The listing builds one solid part. Answer for the finished solid, in the listing's coordinates (mm). A direction names the side the tool comes from. Coordinates: 2 decimals unless noted, no trailing zeros. Loops run counter-clockwise (first coordinate to the right, second up) from the corner with the lowest first, then second, coordinate; pieces in that order, holes last. Notation, with made-up numbers: (53, 87) - (97, 87) arc R38 ccw to (97, 125) - close; hole circle Ø7 at (26.5, -6.5). An arc over 180 degrees is marked (long way). One line per question, with ' | ' between items.
from build123d import *

# Parameters (mm, degrees)
F0_W     = 396.875
F0_H     = 193.675
F1_DEPTH = 193.675
F3_DEPTH = 396.875
F5_R     = 1.45288
F6_DEPTH = 161.925


with BuildPart() as f1:
    # F0 (on Top) → F1 (new body)
    with BuildSketch(Plane.XY):
        with Locations((198.4375, -96.8375)):
            Rectangle(F0_W, F0_H)
        with BuildLine():
            ThreePointArc((31.75, -50.8), (37.329616, -37.329616), (50.8, -31.75))
            Line((50.8, -31.75), (166.6875, -31.75))
            ThreePointArc((166.6875, -31.75), (180.157884, -37.329616), (185.7375, -50.8))
            Line((185.7375, -50.8), (185.7375, -142.875))
            ThreePointArc((185.7375, -142.875), (180.157884, -156.345384), (166.6875, -161.925))
            Line((166.6875, -161.925), (50.8, -161.925))
            ThreePointArc((50.8, -161.925), (37.329616, -156.345384), (31.75, -142.875))
            Line((31.75, -142.875), (31.75, -50.8))
        make_face(mode=Mode.SUBTRACT)
        with BuildLine():
            ThreePointArc((365.125, -142.875), (359.545384, -156.345384), (346.075, -161.925))
            Line((346.075, -161.925), (230.1875, -161.925))
            ThreePointArc((230.1875, -161.925), (216.717116, -156.345384), (211.1375, -142.875))
            Line((211.1375, -142.875), (211.1375, -50.8))
            ThreePointArc((211.1375, -50.8), (216.717116, -37.329616), (230.1875, -31.75))
            Line((230.1875, -31.75), (346.075, -31.75))
            ThreePointArc((346.075, -31.75), (359.545384, -37.329616), (365.125, -50.8))
            Line((365.125, -50.8), (365.125, -142.875))
        make_face(mode=Mode.SUBTRACT)
    extrude(amount=F1_DEPTH)

    # F2 (on face) → F3 (cut)
    with BuildSketch(Plane.YZ.offset(396.875)):
        with BuildLine():
            ThreePointArc((-179.25288, 193.675), (-177.8, 192.22212), (-176.34712, 193.675))
            Line((-176.34712, 193.675), (-179.25288, 193.675))
        make_face()
        with BuildLine():
            Line((-179.25288, 193.675), (-176.34712, 193.675))
            ThreePointArc((-176.34712, 193.675), (-177.8, 195.12788), (-179.25288, 193.675))
        make_face()
        with BuildLine():
            ThreePointArc((-17.32788, 193.675), (-15.875, 192.22212), (-14.42212, 193.675))
            Line((-14.42212, 193.675), (-17.32788, 193.675))
        make_face()
        with BuildLine():
            Line((-17.32788, 193.675), (-14.42212, 193.675))
            ThreePointArc((-14.42212, 193.675), (-15.875, 195.12788), (-17.32788, 193.675))
        make_face()
        with BuildLine():
            Line((-15.875, 0), (-14.42212, 0))
            ThreePointArc((-14.42212, 0), (-15.875, 1.45288), (-17.32788, 0))
            Line((-17.32788, 0), (-15.875, 0))
        make_face()
        with BuildLine():
            ThreePointArc((-17.32788, 0), (-15.875, -1.45288), (-14.42212, 0))
            Line((-14.42212, 0), (-15.875, 0))
            Line((-15.875, 0), (-17.32788, 0))
        make_face()
        with BuildLine():
            Line((-177.8, 0), (-176.34712, 0))
            ThreePointArc((-176.34712, 0), (-177.8, 1.45288), (-179.25288, 0))
            Line((-179.25288, 0), (-177.8, 0))
        make_face()
        with BuildLine():
            ThreePointArc((-179.25288, 0), (-177.8, -1.45288), (-176.34712, 0))
            Line((-176.34712, 0), (-177.8, 0))
            Line((-177.8, 0), (-179.25288, 0))
        make_face()
    extrude(amount=-F3_DEPTH, mode=Mode.SUBTRACT)

    # F5 (on offset) → F6 (cut)
    with BuildSketch(Plane.XZ.offset(15.875)):
        with BuildLine():
            ThreePointArc((196.98462, 193.675), (198.4375, 192.22212), (199.89038, 193.675))
            ThreePointArc((199.89038, 193.675), (198.4375, 195.12788), (196.98462, 193.675))
        make_face()
        with Locations((198.4375, 0)):
            Circle(F5_R)
    extrude(amount=F6_DEPTH, mode=Mode.SUBTRACT)


solid = f1.part
Item 1: Find section A-A, the plane x = 237.5. Write down the section's boundary in (y, z) (3 decimals).
Taken from the geometry:
outline: (-193.675, 0) - (-179.253, 0) arc R1.453 cw to (-176.347, 0) - (-161.925, 0) - (-161.925, 193.675) - (-176.347, 193.675) arc R1.453 cw to (-179.253, 193.675) - (-193.675, 193.675) - close; (-31.75, 0) - (-17.328, 0) arc R1.453 cw to (-14.422, 0) - (0, 0) - (0, 193.675) - (-14.422, 193.675) arc R1.453 cw to (-17.328, 193.675) - (-31.75, 193.675) - close
Item 2: Which of the six approach directions +Z, -Z, +X, -X, +Y, -Y give full straight-line access (tool end or side, diameter ignored) to faces 1 (the face through (196, -7, 193.675)), 2 (the face through (185.738, -96, 95))?
Taken from the geometry:
face 1: +Z, +X, -X, +Y, -Y | face 2: +Z, -Z
Item 3: Find the intervals of material crossed by line 1 (Y direction, x = 158.5, z = 183.5) (3 decimals); line 2 (X direction, y = -48, z = 183.5) (3 decimals); line 3 (X direction, y = -44, z = 160) (3 decimals), in increasing order. Write a range as [from, to].
Taken from the geometry:
line 1: y = [-193.675, -161.925], [-31.75, 0] | line 2: x = [0, 31.957], [185.531, 211.344], [364.918, 396.875] | line 3: x = [0, 33.005], [184.483, 212.392], [363.87, 396.875]
Item 4: The mould has two halves that part along X. Classify faces 3 (the face through (0, -98, 95)), 4 (the face through (180.3, -156.2, 95.5)), 5 (the face through (297, -166, 0)): pulls with the +X half, pulls with the -X half, needs draft (parallel to the pull), parting line crosses it, or undercut.
Taken from the geometry:
face 3: pulls with the -X half | face 4: undercut | face 5: needs draft
Item 5: Find section B-B, the plane y = -57.5. State how many separate pieces and enclosed holes the cut face has, plus the area to 3 significant figures.
Taken from the geometry:
separate pieces: 3 | enclosed holes: 0 | area: 17,200 mm2
